from build123d import *

# Parameters (mm, degrees)
AUFSATZ_LINEAR_AUSTRAGEN1_DEPTH = 10
SCHNITT_LINEAR_AUSTRAGEN1_DEPTH = 21


with BuildPart() as part:
    # Skizze1 → Aufsatz-Linear austragen1 (new body, symmetric)
    with BuildSketch(Plane.XY):
        Polygon((0, 0), (0, 100), (200, 50), (200, 0), align=None)
    extrude(amount=AUFSATZ_LINEAR_AUSTRAGEN1_DEPTH, both=True)

    # Skizze2 → Schnitt-Linear austragen1 (cut, through all)
    with BuildSketch(Plane.XY.offset(10)):
        with BuildLine():
            Line((15, 25), (15, 75))
            ThreePointArc((15, 75), (20, 80), (25, 75))
            Line((25, 75), (25, 25))
            ThreePointArc((25, 25), (20, 20), (15, 25))
        make_face()
    extrude(amount=-SCHNITT_LINEAR_AUSTRAGEN1_DEPTH, mode=Mode.SUBTRACT)


solid = part.part
Geometry: final body of the model. Coordinates: model frame, mm. A direction names the side the tool comes from. Give positions to 0.01 mm unless a question says otherwise; leave off trailing zeros. Loops run counter-clockwise (first coordinate to the right, second up) from the corner with the lowest first, then second, coordinate; pieces in that order, holes last. Notation, with made-up numbers: M 19,31 L 49,31 A16 ccw 49,42 Z; hole C 4,42 d7. An arc over 180 degrees is marked long. Put each result on its own line as item: value. Start each with the question number.
1) Contact query for a flat-ended pin moving along its axis: pin 1 (4 mm diameter, centred on x = 114.5, z = 2, fed in from -Y). Output: stop coordinate, or through.
2) Cut plane D-D (y = 89). Output: boundary loops of the cut face in (x, z), then the cut area to 3 significant figures.
3) Pull-direction query (Y, two-part tool) for faces 1 (the cylindrical face through (20, 20, 0)), 2 (the flat face through (98.6, 75.35, 0.14)), 3 (the flat face through (101, 40, -10)); classes: pulls with the +Y half, pulls with the -Y half, needs draft (parallel to the pull), parting line crosses it, or undercut.
4) Cut plane A-A (y = 69). Output: boundary loops of the cut face in (x, z).
5) Cut plane C-C (z = -4). Output: boundary loops of the cut face in (x, y), then the cut area to 3 significant figures.
6) Ray query, line 1 along X through (y, z) = (29, 3.5); line 2 along Y through (x, z) = (156.5, -8) (3 decimals); line 3 along Y through (x, z) = (108.5, -1.25) (3 decimals). Return the intervals inside material, ascending.
7) Cut plane B-B (x = 20). Output: boundary loops of the cut face in (y, z).
8) Access query for faces 4 (the flat face through (0, 49, 0)), 5 (the flat face through (25, 50, 0)). Directions: +Z, -Z, +X, -X, +Y, -Y. A direction counts if a zero-diameter tool reaches every point of the face in a straight line with its end or side. Return the directions, or none.
Verdict:
1. pin 1: y = 0
2. outline: M 0,-10 L 44,-10 L 44,10 L 0,10 Z
2. area: 880 mm2
3. face 1: undercut
3. face 2: pulls with the +Y half
3. face 3: needs draft
4. outline: M 0,-10 L 15,-10 L 15,10 L 0,10 Z; M 25,-10 L 124,-10 L 124,10 L 25,10 Z
5. outline: M 0,0 L 200,0 L 200,50 L 0,100 Z; hole M 15,25 A5 ccw 25,25 L 25,75 A5 ccw 15,75 Z
5. area: 14,400 mm2
6. line 1: 0 to 15, 25 to 200
6. line 2: 0 to 60.875
6. line 3: 0 to 72.875
7. outline: M 0,-10 L 20,-10 L 20,10 L 0,10 Z; M 80,-10 L 95,-10 L 95,10 L 80,10 Z
8. face 4: +Z, -Z, -X, +Y, -Y
8. face 5: +Z, -Z
